from build123d import *

# Parameters (mm, degrees)
BOSS_EXTRUDE1_DEPTH = 76.2
FILLET1_RADIUS      = 38.1
FILLET1_LENGTH      = 12.7
FILLET2_RADIUS      = 38.1
FILLET2_LENGTH      = 12.7
LPATTERN1_COUNT     = 3
LPATTERN1_PITCH     = 38.1


with BuildPart() as part:
    # Sketch2 → Boss-Extrude1 (new body)
    with BuildSketch(Plane(origin=(0, 0, 0), x_dir=(0, 0, -1), z_dir=(1, 0, 0))):
        with BuildLine():
            Line((-263.244610179, 0), (-182.686659148, 0))
            ThreePointArc((-182.686659148, 0), (-163.246340784, 3.866919748), (-146.765634664, 14.878975516))
            Line((-146.765634664, 14.878975516), (146.765634664, 308.410244843))
            ThreePointArc((146.765634664, 308.410244843), (163.246340784, 319.42230061), (182.686659148, 323.289220358))
            Line((182.686659148, 323.289220358), (339.444610179, 323.289220358))
            Line((339.444610179, 323.289220358), (339.444610179, 310.589220358))
            Line((339.444610179, 310.589220358), (182.686659148, 310.589220358))
            ThreePointArc((182.686659148, 310.589220358), (168.106420375, 307.689030547), (155.745890785, 299.429988722))
            Line((155.745890785, 299.429988722), (-137.785378542, 5.898719395))
            ThreePointArc((-137.785378542, 5.898719395), (-158.386261193, -7.866350314), (-182.686659148, -12.7))
            Line((-182.686659148, -12.7), (-263.244610179, -12.7))
            Line((-263.244610179, -12.7), (-263.244610179, 0))
        make_face()
    extrude(amount=BOSS_EXTRUDE1_DEPTH)

    # Fillet1: full round fillet: the end face becomes a half cylinder, R = half its width
    fillet1_face = Plane((38.1, -6.35, 263.244610179), x_dir=(0, -1, 0), z_dir=(0, 0, 1))  # on the end face: x along it, z out of the body
    fillet1_slab = fillet1_face.offset(-FILLET1_RADIUS / 2) * Box(FILLET1_LENGTH, 2 * FILLET1_RADIUS, FILLET1_RADIUS, mode=Mode.PRIVATE)  # the body's end, R deep
    fillet1_round = Plane((38.1, -6.35, 225.144610179), x_dir=(0, 0, 1), z_dir=(0, -1, 0)) * Cylinder(FILLET1_RADIUS, FILLET1_LENGTH, mode=Mode.PRIVATE)  # its axis R under the face
    add(fillet1_slab - fillet1_round, mode=Mode.SUBTRACT)

    # Fillet2: full round fillet: the end face becomes a half cylinder, R = half its width
    fillet2_face = Plane((38.1, 316.939220358, -339.444610179), x_dir=(0, 1, 0), z_dir=(0, 0, -1))  # on the end face: x along it, z out of the body
    fillet2_slab = fillet2_face.offset(-FILLET2_RADIUS / 2) * Box(FILLET2_LENGTH, 2 * FILLET2_RADIUS, FILLET2_RADIUS, mode=Mode.PRIVATE)  # the body's end, R deep
    fillet2_round = Plane((38.1, 316.939220358, -301.344610179), x_dir=(0, 0, -1), z_dir=(0, 1, 0)) * Cylinder(FILLET2_RADIUS, FILLET2_LENGTH, mode=Mode.PRIVATE)  # its axis R under the face
    add(fillet2_slab - fillet2_round, mode=Mode.SUBTRACT)

    # Sketch4 → 1 (1) Diameter Hole1 (revolve, cut)
    with BuildSketch(Plane(origin=(38.1, 0, 225.144610179), x_dir=(0, 0, 1), z_dir=(1, 0, 0))):
        Polygon((0, 0), (0, 12.7), (12.7, 12.7), (12.7, 0.635), (13.335, 0), align=None)
    revolve(axis=Axis((38.1, 6.35, 225.144610179), (0, -1, 0)), mode=Mode.SUBTRACT)

    # Sketch7 → 1 (1) Diameter Hole2 (revolve, cut)
    with BuildSketch(Plane(origin=(38.1, 310.589220358, -301.344610179), x_dir=(0, 0, -1), z_dir=(1, 0, 0))):
        Polygon((0, 0), (0, 12.7), (12.7, 12.7), (12.7, 0.635), (13.335, 0), align=None)
    f_1_1_diameter_hole2 = revolve(axis=Axis((38.1, 304.239220358, -301.344610179), (0, 1, 0)), mode=Mode.SUBTRACT)

    # LPattern1: 1 (1) Diameter Hole2 ×3
    with Locations(*[(0, 0, i * LPATTERN1_PITCH) for i in range(1, LPATTERN1_COUNT)]):
        add(f_1_1_diameter_hole2, mode=Mode.SUBTRACT)


solid = part.part
Can you work these out from the model? Positions are in its coordinate system, mm. A direction names the side the tool comes from. Give positions to 0.01 mm unless a question says otherwise; leave off trailing zeros. Loops run counter-clockwise (first coordinate to the right, second up) from the corner with the lowest first, then second, coordinate; pieces in that order, holes last. Notation, with made-up numbers: (73, 36) -> (104, 36) arc R8 ccw to (104, 46) -> close; hole circle Ø4 at (57, -7). An arc over 180 degrees is marked (long way). Return JSON: item names as keys, results as strings.
Q1. I want a section at A-A, the plane x = 58. List the corners of the cut face in (y, z) for me.
Checks:
{"outline": "(-12.7, 182.69) arc R63.5 ccw to (5.9, 137.79) -> (299.43, -155.75) arc R38.1 cw to (310.59, -182.69) -> (310.59, -333.83) -> (323.29, -333.83) -> (323.29, -182.69) arc R50.8 ccw to (308.41, -146.77) -> (14.88, 146.77) arc R50.8 cw to (0, 182.69) -> (0, 257.63) -> (-12.7, 257.63) -> close"}
Q2. I want a section at C-C, the plane y = 175. List the corners of the cut face in (x, z) for me, then the cut area to 3 significant figures.
Checks:
{"outline": "(0, -31.32) -> (76.2, -31.32) -> (76.2, -13.36) -> (0, -13.36) -> close", "area": "1,370 mm2"}
Q3. I need wall thicknesses on probe 1 along Z at (x, y) = (38.1, 314); probe 2 along Z at (x, y) = (38.1, 314.5); probe 3 along Y at (x, z) = (8, -258.5). Which ranges of each line are inside material? Lowest first, please.
Checks:
{"probe 1": "z = -339.44 to -314.04, -288.64 to -275.94, -250.54 to -237.84, -212.44 to -153.4", "probe 2": "z = -339.44 to -314.04, -288.64 to -275.94, -250.54 to -237.84, -212.44 to -154.13", "probe 3": "y = 310.59 to 323.29"}
Q4. For pin 1 Ø10 at (x, z) = (48.5, -50) entering from +Y; pin 2 Ø23 at (x, z) = (34.5, -269) entering from -Y; pin 3 Ø20.5 at (x, z) = (38.1, -263.24) entering from -Y; pin 4 Ø10 at (x, z) = (65.5, -67) entering from -Y, each with a flat end and sliding along its axis, tell me the tip position at first contact or that it passes through.
Checks:
{"pin 1": "stops at y = 216.64", "pin 2": "stops at y = 310.59", "pin 3": "passes through", "pin 4": "stops at y = 205.68"}
Q5. I want a section at B-B, the plane z = 193. List the corners of the cut face in (x, y) for me, then the cut area to 3 significant figures.
Checks:
{"outline": "(0, -12.7) -> (76.2, -12.7) -> (76.2, 0) -> (0, 0) -> close", "area": "968 mm2"}
Q6. We'd pull the mould along X, two halves only. Please class faces 1 (the face through (42.96, -6.58, 236.88)), 2 (the face through (38.938, -6.439, 263.235)), 3 (the face through (37.57, -7.73, 158.06)), 4 (the face through (76.2, 169, -20)): released by +X, released by -X, zero draft, split by the parting line, or undercut.
Checks:
{"face 1": "undercut", "face 2": "split by the parting line", "face 3": "zero draft", "face 4": "released by +X"}
Q7. On a 3-axis mill with a long thin cutter (end or side, diameter ignored), from which of +Z, -Z, +X, -X, +Y, -Y can I reach the whole of each face in a straight line? I mean faces 5 (the face through (38, 310.589, -245)), 6 (the face through (29, 0, 215)), 7 (the face through (38, 323.289, -243)). Say none if no direction works.
Checks:
{"face 5": "-Z, +X, -X, -Y", "face 6": "+Z, +X, -X, +Y", "face 7": "+Z, -Z, +X, -X, +Y"}
